Source: CAD feature listing. Evaluate the final solid. Frame: model axes, mm. A direction names the side the tool comes from. Round coordinates to 2 decimals unless told otherwise and drop trailing zeros. Order: outer loops, then holes, each group sorted by start corner. A loop starts at its lowest first (then second) coordinate and runs counter-clockwise, first axis right, second up. Notation, with made-up numbers: M -3,-25.5 L 5,-25.5 A35 ccw 5,9.5 Z; hole C 38.25,50 d4. An arc over 180 degrees is marked long. Use one line per item in the form item = value. Start each with the question number.
Q1. Material intervals for probe 1 along X at (y, z) = (-24, 53.5); probe 2 along Y at (x, z) = (-78.5, 72); probe 3 along Y at (x, z) = (18.5, 32.5), sorted ascending.
Q2. Pull-direction query (Y, two-part tool) for faces 3 (the flat face through (198.438, -1, 1)), 4 (the flat face through (-3, 96.838, 1)), 5 (the flat face through (-89, -65.088, 1)); classes: pulls with the +Y half, pulls with the -Y half, needs draft (parallel to the pull), parting line crosses it, or undercut.
Q3. Reachability of faces 1 (the flat face through (-3, 1, 96.838)), 2 (the cylindrical face through (161.914, 60.561, 1.356)) from +Z, -Z, +X, -X, +Y, -Y: full face, straight path, thin tool, end or side. Return the list, or none.
Q4. Section A-A (x = -75). Return the cut outline in (y, z), plus the area to 3 significant figures.
Q5. Section B-B (y = 17). Return the cut outline in (x, z).
Q6. Section C-C (z = -34.5). Give the number of separate pieces and of enclosed holes in the cut face, plus the area to 3 significant figures.
Q7. Section D-D (y = 56). Return the cut outline in (x, z), plus the area to 3 significant figures.
Q8. Contact query for a flat-ended pin moving along its axis: pin 1 (6 mm diameter, centred on x = 16.5, y = 36, fed in from +Z). Output: stop coordinate, or through.
from build123d import *

# Parameters (mm, degrees)
F0_W     = 396.875
F0_H     = 193.675
F1_DEPTH = 96.8375


with BuildPart() as f1:
    # F0 (on Top) → F1 (new body, symmetric)
    with BuildSketch(Plane.XY):
        Rectangle(F0_W, F0_H)
        with BuildLine():
            ThreePointArc((-166.6875, 49.2125), (-162.03782, 60.43782), (-150.8125, 65.0875))
            Line((-150.8125, 65.0875), (-28.575, 65.0875))
            ThreePointArc((-28.575, 65.0875), (-17.34968, 60.43782), (-12.7, 49.2125))
            Line((-12.7, 49.2125), (-12.7, 0))
            Line((-12.7, 0), (-12.7, -49.2125))
            ThreePointArc((-12.7, -49.2125), (-17.34968, -60.43782), (-28.575, -65.0875))
            Line((-28.575, -65.0875), (-150.8125, -65.0875))
            ThreePointArc((-150.8125, -65.0875), (-162.03782, -60.43782), (-166.6875, -49.2125))
            Line((-166.6875, -49.2125), (-166.6875, 49.2125))
        make_face(mode=Mode.SUBTRACT)
        with BuildLine():
            Line((12.7, -49.2125), (12.7, 0))
            Line((12.7, 0), (12.7, 49.2125))
            ThreePointArc((12.7, 49.2125), (17.34968, 60.43782), (28.575, 65.0875))
            Line((28.575, 65.0875), (150.8125, 65.0875))
            ThreePointArc((150.8125, 65.0875), (162.03782, 60.43782), (166.6875, 49.2125))
            Line((166.6875, 49.2125), (166.6875, -49.2125))
            ThreePointArc((166.6875, -49.2125), (162.03782, -60.43782), (150.8125, -65.0875))
            Line((150.8125, -65.0875), (28.575, -65.0875))
            ThreePointArc((28.575, -65.0875), (17.34968, -60.43782), (12.7, -49.2125))
        make_face(mode=Mode.SUBTRACT)
    extrude(amount=F1_DEPTH, both=True)


solid = f1.part
Results list:
q1.probe_1 = -198.44 to -166.69, -12.7 to 12.7, 166.69 to 198.44
q1.probe_2 = -96.84 to -65.09, 65.09 to 96.84
q1.probe_3 = -96.84 to -61.48, 61.48 to 96.84
q2.face_3 = needs draft
q2.face_4 = pulls with the +Y half
q2.face_5 = undercut
q3.face_1 = +Z, +X, -X, +Y, -Y
q3.face_2 = +Z, -Z
q4.outline = M -96.84,-96.84 L -65.09,-96.84 L -65.09,96.84 L -96.84,96.84 Z; M 65.09,-96.84 L 96.84,-96.84 L 96.84,96.84 L 65.09,96.84 Z
q4.area = 12,300 mm2
q5.outline = M -198.44,-96.84 L -166.69,-96.84 L -166.69,96.84 L -198.44,96.84 Z; M -12.7,-96.84 L 12.7,-96.84 L 12.7,96.84 L -12.7,96.84 Z; M 166.69,-96.84 L 198.44,-96.84 L 198.44,96.84 L 166.69,96.84 Z
q6.separate_pieces = 1
q6.enclosed_holes = 2
q6.area = 37,200 mm2
q7.outline = M -198.44,-96.84 L -165.16,-96.84 L -165.16,96.84 L -198.44,96.84 Z; M -14.22,-96.84 L 14.22,-96.84 L 14.22,96.84 L -14.22,96.84 Z; M 165.16,-96.84 L 198.44,-96.84 L 198.44,96.84 L 165.16,96.84 Z
q7.area = 18,400 mm2
q8.pin_1 = through
